Build history of the part. All positions in model axes, mm. Coordinates: 2 decimals unless noted, no trailing zeros. Write each loop counter-clockwise with the first axis right and the second up, starting at its lowest first coordinate (ties: lowest second). Pieces come first, ordered by that corner, then holes. Notation, with made-up numbers: (76, 58) -> (84, 58) arc R6 ccw to (84, 67) -> close; hole circle Ø8 at (-37.5, 45). An arc over 180 degrees is marked (long way). Write each question's results on one line, items separated by ' | '. Start each with the question number.
Q1. Saw through at A-A on z = -13. Give the cut face in (x, y).
Q2. Drill centre lines: line 1 (X direction, y = 242.5, z = -12.5); line 2 (X direction, y = -9.5, z = -327); line 3 (Z direction, x = 257, y = -94). Where is each one in solid material? Low to high.
Q3. Drop flat-ended pins along their axis: pin 1 Ø10 at (x, y) = (229, 155.5) entering from -Z; pin 2 Ø2 at (y, z) = (-62, 212) entering from +X. Give the stop position or say it passes through.
from build123d import *

# Parameters (mm, degrees)
BOSS_EXTRUDE1_DEPTH = 490
FILLET1_R           = 100


with BuildPart() as part:
    # Sketch1 → Boss-Extrude1 (new, symmetric)
    with BuildSketch(Plane.XY):
        Polygon((0, 550), (0, -550), (350, -550), (350, -270), (200, 550), align=None)
    extrude(amount=BOSS_EXTRUDE1_DEPTH, both=True)

    # Fillet1
    fillet1_edges = [part.edges().sort_by_distance(p)[0] for p in [
        (350, -410, 490),
        (275, 140, 490),
        (275, 140, -490),
        (350, -410, -490),
        (200, 550, 0),
        (350, -270, 0),
        (350, -550, 0),
    ]]
    fillet(fillet1_edges, radius=FILLET1_R)


solid = part.part
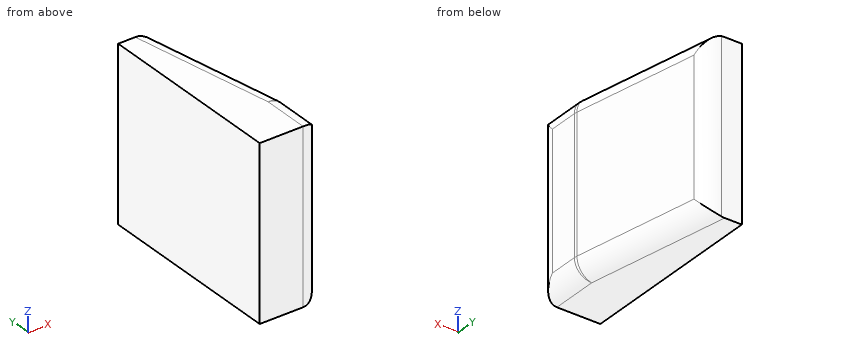
Returned:
1) outline: (0, -550) -> (250, -550) arc R100 ccw to (350, -450) -> (350, -279.07) arc R100 ccw to (348.37, -261.08) -> (215, 467.99) arc R100 ccw to (116.63, 550) -> (0, 550) -> close
2) line 1: x = 0 to 256.25 | line 2: x = 0 to 302.35 | line 3: z = -481.57 to 481.57
3) pin 1: stops at z = -475.09 | pin 2: stops at x = 312.13
